Source: three-view drawing plus pictorial views. Frame: mm from the lowest corner of the part. A direction names the side the tool comes from. Round coordinates to 2 decimals unless told otherwise and drop trailing zeros. Loops run counter-clockwise (first coordinate to the right, second up) from the corner with the lowest first, then second, coordinate; pieces in that order, holes last. Notation, with made-up numbers: (22.5, 76.5) -> (50.5, 76.5) arc R36 cw to (50.5, 111.5) -> close; hole circle Ø4 at (25, 79). An arc over 180 degrees is marked (long way). Answer in a Markdown table with one row per item.
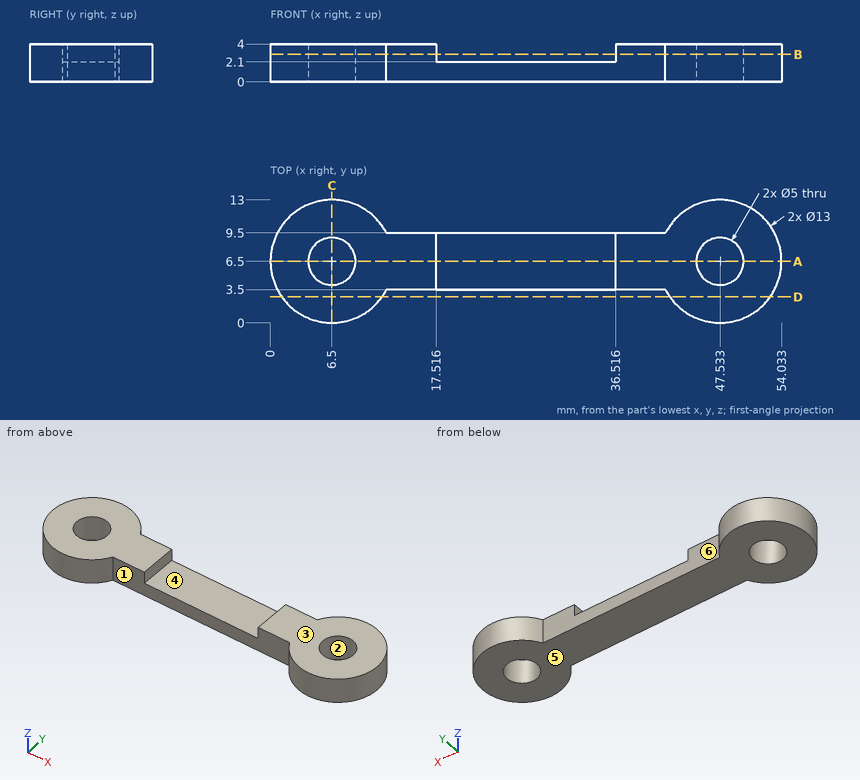
Item 1: Reachability of the marked faces 4, 5 and 6 from +Z, -Z, +X, -X, +Y, -Y: full face, straight path, thin tool, end or side. Return the list, or none.
Answer:
| item | result |
|---|---|
| face 4 | +Z, +Y, -Y |
| face 5 | -Z, +X, -X, +Y, -Y |
| face 6 | +Z, -Z, +Y |
Item 2: Cut plane A-A (y = 6.5). Output: boundary loops of the cut face in (x, z), then the cut area to 3 significant figures.
Answer:
| item | result |
|---|---|
| outline | (0, 0) -> (4, 0) -> (4, 4) -> (0, 4) -> close; (9, 0) -> (45.03, 0) -> (45.03, 4) -> (36.52, 4) -> (36.52, 2.1) -> (17.52, 2.1) -> (17.52, 4) -> (9, 4) -> close; (50.03, 0) -> (54.03, 0) -> (54.03, 4) -> (50.03, 4) -> close |
| area | 140 mm² |
Item 3: Draft query along Y for the marked faces 1, 2 and 3. Return one class per face: pulls with the +Y half, pulls with the -Y half, needs draft (parallel to the pull), parting line crosses it, or undercut.
Answer:
| item | result |
|---|---|
| face 1 | pulls with the -Y half |
| face 2 | undercut |
| face 3 | needs draft |
Item 4: Line query: probe 1 along X at (y, z) = (6.5, 2.8); probe 2 along X at (y, z) = (6.75, 0.5) (1 decimal); probe 3 along X at (y, z) = (8.25, 2.3) (1 decimal). Output: solid intervals per line, ascending. Write a range as [from, to].
Answer:
| item | result |
|---|---|
| probe 1 | x = [0, 4], [9, 17.52], [36.52, 45.03], [50.03, 54.03] |
| probe 2 | x = [0, 4], [9, 45], [50, 54] |
| probe 3 | x = [0.2, 4.7], [8.3, 17.5], [36.5, 45.7], [49.3, 53.8] |
Item 5: Cut plane D-D (y = 2.75). Output: boundary loops of the cut face in (x, z).
Answer:
| item | result |
|---|---|
| outline | (1.19, 0) -> (11.81, 0) -> (11.81, 4) -> (1.19, 4) -> close; (42.22, 0) -> (52.84, 0) -> (52.84, 4) -> (42.22, 4) -> close |
Item 6: Cut plane C-C (x = 6.5). Output: boundary loops of the cut face in (y, z).
Answer:
| item | result |
|---|---|
| outline | (0, 0) -> (4, 0) -> (4, 4) -> (0, 4) -> close; (9, 0) -> (13, 0) -> (13, 4) -> (9, 4) -> close |
Item 7: Pin query (flat end, axial travel): pin 1 Ø2 at (x, z) = (28, 3) entering from -Y; pin 2 Ø6.5 at (x, y) = (6.5, 6.5) entering from +Z; pin 3 Ø0.6 at (y, z) = (6, 3) entering from -X; pin 4 Ø1.5 at (y, z) = (5, 3) entering from +X. Return the tip coordinate at first contact, or that it passes through.
Answer:
| item | result |
|---|---|
| pin 1 | stops at y = 3.5 |
| pin 2 | stops at z = 4 |
| pin 3 | stops at x = 0 |
| pin 4 | stops at x = 53.99 |
Item 8: Cut plane B-B (z = 2.9). Output: boundary loops of the cut face in (x, y), then the cut area to 3 significant figures.
Answer:
| item | result |
|---|---|
| outline | (12.27, 3.5) -> (17.52, 3.5) -> (17.52, 9.5) -> (12.27, 9.5) arc R6.5 ccw (long way) to start; (36.52, 3.5) -> (41.77, 3.5) arc R6.5 ccw (long way) to (41.77, 9.5) -> (36.52, 9.5) -> close; hole circle Ø5 at (6.5, 6.5); hole circle Ø5 at (47.53, 6.5) |
| area | 283 mm² |
